For this review, take the finished solid that the model builds, in its own axes (mm). A direction names the side the tool comes from. Coordinates: 2 decimals unless noted, no trailing zeros. Loops run counter-clockwise (first coordinate to the right, second up) from the corner with the lowest first, then second, coordinate; pieces in that order, holes last. Notation, with made-up numbers: (35, 25) - (67, 25) arc R19 cw to (67, 35) - close; hole circle Ø5 at (86, 80.25). An arc over 180 degrees is marked (long way). Answer as a JSON object with one key per item and string values. Group by question number.
Item 1: Mouldability with a two-part tool opening along X and no side actions: class faces 1 (the flat face through (-3.03, -6.02, 4.43)), 2 (the flat face through (-46, 18.05, 1)), 3 (the cylindrical face through (49.64, -29.16, 1.48)) as released by +X, released by -X, zero draft, split by the parting line, or undercut.
Item 2: We need section D-D (y = -19.5). Give the boundary of the cut face in (x, z).
Item 3: Clearance check with flat-ended pins moving along their axes: pin 1 (1.5 mm diameter, centred on x = -36.5, z = 5, fed in from -Y); pin 2 (2.5 mm diameter, centred on x = -35.5, z = 3.5, fed in from +Y); pin 3 (1.5 mm diameter, centred on x = -48, z = 2, fed in from -Y); pin 4 (0.9 mm diameter, centred on x = 36.5, z = 5, fed in from -Y). State where each tip first meets the part, or that it passes through.
Item 4: We need section A-A (x = 50). Give the boundary of the cut face in (y, z), then the cut area to 3 significant figures.
Item 5: Tool access review of faces 4 (the flat face through (-33, 33.95, 4)), 5 (the flat face through (33, -33.95, 4)), 6 (the flat face through (-35, 21.15, 4)), 7 (the flat face through (5, 6, 3)): name each direction out of +Z, -Z, +X, -X, +Y, -Y from which nothing blocks a thin tool from reaching the whole face with its end or side.
Item 6: We need section B-B (z = 1.95). Give the boundary of the cut face in (x, y).
Item 7: To check wall thickness, follow line 1 (Y direction, x = -50, z = 2.45); line 2 (Y direction, x = 50, z = 1.1); line 3 (Z direction, x = 2.5, y = 10). State the ranges of each line that lie inside material, in increasing order.
from build123d import *

# Parameters (mm, degrees)
SKETCH_1_R      = 1.65
EXTRUDE_1_DEPTH = 3
EXTRUDE_2_DEPTH = 2.9
CHAMFER_1_SIZE  = 2.9
FILLET_1_R      = 1


with BuildPart() as part:
    # 草图1 → 凸台-拉伸1 (new body)
    with BuildSketch(Plane.XY):
        Polygon((-60, 37.05), (-23.614971157, 37.05), (31.485028843, -18.05), (60, -18.05), (60, -37.05), (23.614971157, -37.05), (-31.485028843, 18.05), (-60, 18.05), align=None)
        with Locations((-50, 27.55)):
            Circle(SKETCH_1_R, mode=Mode.SUBTRACT)
        with Locations((50, -27.55)):
            Circle(SKETCH_1_R, mode=Mode.SUBTRACT)
    extrude(amount=EXTRUDE_1_DEPTH)

    # 草图2 → 凸台-拉伸2 (add)
    with BuildSketch(Plane.XY.offset(3)):
        Polygon((-41, 33.95), (-41, 21.15), (-30.200966799, 21.15), (24.899033201, -33.95), (41, -33.95), (41, -21.15), (30.200966799, -21.15), (-24.899033201, 33.95), align=None)
    extrude(amount=EXTRUDE_2_DEPTH)

    # 倒角1
    chamfer_1_edges = [part.edges().sort_by_distance(p)[0] for p in [
        (41, -27.55, 5.9),
        (-41, 27.55, 5.9),
    ]]
    chamfer(chamfer_1_edges, length=CHAMFER_1_SIZE - 0.0001)  # a hair under: the kernel refuses the full size

    # 圆角1
    fillet_1_edges = [part.edges().sort_by_distance(p)[0] for p in [
        (-23.614971157, 37.05, 1.5),
        (31.485028843, -18.05, 1.5),
        (23.614971157, -37.05, 1.5),
        (-31.485028843, 18.05, 1.5),
        (-24.899033201, 33.95, 4.45),
        (-30.200966799, 21.15, 4.45),
        (24.899033201, -33.95, 4.45),
        (30.200966799, -21.15, 4.45),
    ]]
    fillet(fillet_1_edges, radius=FILLET_1_R)


solid = part.part
Check sheet entries:
{
 "1": {"face 1": "released by -X", "face 2": "zero draft", "face 3": "undercut"},
 "2": {"outline": "(6.06, 0) - (60, 0) - (60, 3) - (28.55, 3) - (28.55, 5.9) - (10.45, 5.9) - (10.45, 3) - (6.06, 3) - close"},
 "3": {"pin 1": "stops at y = 21.15", "pin 2": "stops at y = 37.05", "pin 3": "stops at y = 18.05", "pin 4": "stops at y = -33.95"},
 "4": {"outline": "(-37.05, 0) - (-29.2, 0) - (-29.2, 3) - (-37.05, 3) - close; (-25.9, 0) - (-18.05, 0) - (-18.05, 3) - (-25.9, 3) - close", "area": "47.1 mm2"},
 "5": {"face 4": "+Z, +X, -X, +Y", "face 5": "+Z, +X, -X, -Y", "face 6": "+Z, -X, -Y", "face 7": "+Z"},
 "6": {"outline": "(-60, 18.05) - (-31.9, 18.05) arc R1 cw to (-31.19, 17.76) - (23.32, -36.76) arc R1 ccw to (24.03, -37.05) - (60, -37.05) - (60, -18.05) - (31.9, -18.05) arc R1 cw to (31.19, -17.76) - (-23.32, 36.76) arc R1 ccw to (-24.03, 37.05) - (-60, 37.05) - close; hole circle Ø3.3 at (-50, 27.55); hole circle Ø3.3 at (50, -27.55)"},
 "7": {"line 1": "y = 18.05 to 25.9, 29.2 to 37.05", "line 2": "y = -37.05 to -29.2, -25.9 to -18.05", "line 3": "z = 0 to 3"}
}
